```python
from build123d import *

# Parameters (mm, degrees)
SKETCH1_R                 = 11.5
BOSS_EXTRUDE1_DEPTH       = 1.45
BOSS_EXTRUDE2_DEPTH       = 1.45
CIRPATTERN2_COUNT         = 5
SKETCH4_R                 = 4
CUT_EXTRUDE1_DEPTH        = 1.45
BOSS_EXTRUDE3_START       = 5
SKETCH5_R                 = 7
SKETCH5_R_2               = 4
BOSS_EXTRUDE3_DEPTH       = 5
M2X0_4_TAPPED_HOLE3_D     = 1.6
M2X0_4_TAPPED_HOLE3_DEPTH = 5.2
M2X0_4_TAPPED_HOLE3_TIP   = 0.480688495


with BuildPart() as part:
    # Sketch1 → Boss-Extrude1 (new body)
    with BuildSketch(Plane.XY):
        Circle(SKETCH1_R)
    extrude(amount=BOSS_EXTRUDE1_DEPTH)

    # Sketch2 → Boss-Extrude2 (add)
    with BuildSketch(Plane.XY.offset(1.45)):
        with BuildLine():
            Line((11.466388324, -0.781762992), (11.466388324, 0.781762992))
            ThreePointArc((11.466388324, 0.781762992), (12.435767446, 0.634469665), (13.317644229, 0.205885315))
            ThreePointArc((13.317644229, 0.205885315), (13.425830137, 0), (13.317644229, -0.205885315))
            ThreePointArc((13.317644229, -0.205885315), (12.435767446, -0.634469665), (11.466388324, -0.781762992))
        make_face()
    boss_extrude2 = extrude(amount=-BOSS_EXTRUDE2_DEPTH)

    # CirPattern2: Boss-Extrude2 ×5 about axis
    cirpattern2_axis = Axis((0, 0, 0), (0, 0, 1))
    for i in range(1, CIRPATTERN2_COUNT):
        add(boss_extrude2.rotate(cirpattern2_axis, i * 360 / CIRPATTERN2_COUNT))

    # Sketch4 → Cut-Extrude1 (cut)
    with BuildSketch(Plane.XY.offset(1.45)):
        Circle(SKETCH4_R)
    extrude(amount=-CUT_EXTRUDE1_DEPTH, mode=Mode.SUBTRACT)

    # Sketch5 → Boss-Extrude3 (add)
    with BuildSketch(Plane.XY.offset(1.45).offset(BOSS_EXTRUDE3_START)):
        Circle(SKETCH5_R)
        Circle(SKETCH5_R_2, mode=Mode.SUBTRACT)
    extrude(amount=-BOSS_EXTRUDE3_DEPTH)

    # M2x0.4 Tapped Hole3
    with Locations(Plane(origin=(-0.021974878, 6.999965507, 3.87491846), x_dir=(0.999995072485, 0.003139268242, 0), z_dir=(-0.003139268242, 0.999995072485, 0))):
        with Locations((0, 0)):
            Hole(M2X0_4_TAPPED_HOLE3_D / 2, depth=M2X0_4_TAPPED_HOLE3_DEPTH)
            with Locations((0, 0, -(M2X0_4_TAPPED_HOLE3_DEPTH + M2X0_4_TAPPED_HOLE3_TIP / 2))):  # 118° drill point
                Cone(0, M2X0_4_TAPPED_HOLE3_D / 2, M2X0_4_TAPPED_HOLE3_TIP, mode=Mode.SUBTRACT)


solid = part.part
```
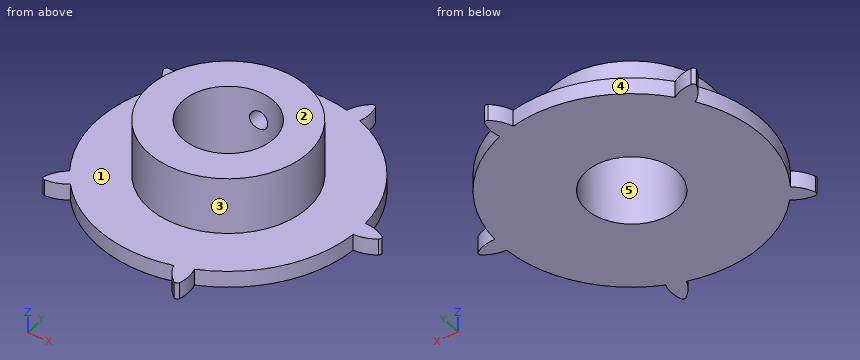
Work out the finished part from the listing and answer in its coordinate system (mm). Face numbers are marked on the shaded views. A direction names the side the tool comes from. Coordinates: 2 decimals unless noted, no trailing zeros. Write each loop counter-clockwise with the first axis right and the second up, starting at its lowest first coordinate (ties: lowest second). Pieces come first, ordered by that corner, then holes. Notation, with made-up numbers: (49, -18) - (106, -18) arc R20 cw to (106, 0) - close; hole circle Ø5 at (58, 60.25). An arc over 180 degrees is marked (long way). Answer as a JSON object with one key per item and string values.
Q1. Which of the six approach directions +Z, -Z, +X, -X, +Y, -Y give full straight-line access (tool end or side, diameter ignored) to the marked faces 1 and 2?
Results list:
{"face 1": "+Z", "face 2": "+Z, +X, -X, +Y, -Y"}
Q2. For a pull along Y with two mould halves and no side action, classify the marked faces 3, 4 and 5 as pulls with the +Y half, pulls with the -Y half, needs draft (parallel to the pull), parting line crosses it, or undercut.
Results list:
{"face 3": "parting line crosses it", "face 4": "pulls with the +Y half", "face 5": "undercut"}
Q3. Find section B-B (z = 5.25). Write down the section's boundary in (x, y).
Results list:
{"outline": "circle Ø14 at (0, 0); hole circle Ø8 at (0, 0)"}
Q4. Consider L1, parallel to Y at x = 0, z = 2; L2, parallel to Z at x = -6.25, y = -8.5; L3, parallel to X at y = -2, z = 5.75. Determine where each line is inside the solid, lowest interval first. Write a range as from..to.
Results list:
{"L1": "y = -7..-4, 4..7", "L2": "z = 0..1.45", "L3": "x = -6.71..-3.46, 3.46..6.71"}
Q5. Find section C-C (x = -4.5). Write down the section's boundary in (y, z), plus the area to 3 significant figures.
Results list:
{"outline": "(-10.58, 0) - (10.58, 0) - (10.58, 1.45) - (5.36, 1.45) - (5.36, 6.45) - (-5.36, 6.45) - (-5.36, 1.45) - (-10.58, 1.45) - close", "area": "84.3 mm^2"}
Q6. Find section D-D (x = 0). State how many separate pieces and enclosed holes the cut face has, plus the area to 3 significant figures.
Results list:
{"separate pieces": "3", "enclosed holes": "0", "area": "47.0 mm^2"}
Q7. Find section A-A (y = -3.5). Write down the section's boundary in (x, z), plus the area to 3 significant figures.
Results list:
{"outline": "(-10.95, 0) - (-1.94, 0) - (-1.94, 6.45) - (-6.06, 6.45) - (-6.06, 1.45) - (-10.95, 1.45) - close; (1.94, 0) - (10.95, 0) - (10.95, 1.45) - (6.06, 1.45) - (6.06, 6.45) - (1.94, 6.45) - close", "area": "67.4 mm^2"}
Q8. Given pin 1 Ø1.5 at (y, z) = (2.5, 4) entering from +X; pin 2 Ø3 at (x, z) = (-2.5, 2.5) entering from +Y, each flat-ended and moving along its own axis, determine where each tip first touches the part or whether it passes through.
Results list:
{"pin 1": "stops at x = 6.78", "pin 2": "stops at y = 11.41"}
